```python
from build123d import *

# Parameters (mm, degrees)
SKETCH1_R           = 40
BOSS_EXTRUDE1_DEPTH = 30
FILLET1_R           = 5
SKETCH2_R           = 36
CUT_EXTRUDE1_DEPTH  = 25


with BuildPart() as part:
    # Sketch1 → Boss-Extrude1 (new body)
    with BuildSketch(Plane(origin=(0, 0, 0), x_dir=(1, 0, 0), z_dir=(0, 1, 0))):
        with Locations(Location((0, 0, 0), (0, 0, 270))):
            Circle(SKETCH1_R)
    extrude(amount=BOSS_EXTRUDE1_DEPTH)

    # Fillet1
    fillet1_edges = [part.edges().sort_by_distance(p)[0] for p in [
        (0, 30, -40),
    ]]
    fillet(fillet1_edges, radius=FILLET1_R)

    # Sketch2 → Cut-Extrude1 (cut)
    with BuildSketch(Plane.XZ):
        with Locations(Location((0, 0, 0), (0, 0, 270))):
            Circle(SKETCH2_R)
    extrude(amount=-CUT_EXTRUDE1_DEPTH, mode=Mode.SUBTRACT)


solid = part.part
```
CAD build for the part. Positions are in the model's coordinates, mm. A direction names the side the tool comes from. Round coordinates to 2 decimals unless told otherwise and drop trailing zeros. Order: outer loops, then holes, each group sorted by start corner. A loop starts at its lowest first (then second) coordinate and runs counter-clockwise, first axis right, second up.
Item 1: Saw through at A-A on z = 0. Write the cut outline in (x, y).
Item 2: Pin check, flat tips, straight feed: pin 1 (4 mm diameter, centred on x = -8.5, y = 24.5, fed in from +Z); pin 2 (5 mm diameter, centred on y = 10, z = 3, fed in from +X); pin 3 (1 mm diameter, centred on x = -15, y = 14, fed in from +Z); pin 4 (6 mm diameter, centred on x = 0, y = 25.5, fed in from +Z). Stop position of each tip, or through.
Item 3: Probe line 1 along X through (y, z) = (19.5, 0); line 2 along Y through (x, z) = (7, 15); line 3 along X through (y, z) = (8.25, -12). List the from-to ranges inside material, lowest first.
Item 4: Saw through at B-B on x = 0. Write the cut outline in (y, z), then the cut area to 3 significant figures.
Item 5: Saw through at C-C on y = 11.25. Write the cut outline in (x, z), then the cut area to 3 significant figures.
Item 6: Saw through at D-D on y = 26.75. Write the cut outline in (x, z), then the cut area to 3 significant figures.
Item 7: Mould opens along X. For faces 3 (the face through (0, 30, 0)), 4 (the face through (1, 25, 1)), 5 (the face through (-39.05, 12.32, -8.67)) say: pulls with the +X half, pulls with the -X half, needs draft (parallel to the pull), parting line crosses it, or undercut.
Item 8: Tool access for faces 1 (the face through (15, 0, -33)), 2 (the face through (10.81, 12.32, -34.34)): list every direction of +Z, -Z, +X, -X, +Y, -Y with a clear straight run to the whole face (end or side of a thin tool).
Reported:
1. outline: (-40, 0) - (-36, 0) - (-36, 25) - (36, 25) - (36, 0) - (40, 0) - (40, 25) arc R5 ccw to (35, 30) - (-35, 30) arc R5 ccw to (-40, 25) - close
2. pin 1: stops at z = 39.47
2. pin 2: stops at x = 40
2. pin 3: stops at z = 37.28
2. pin 4: stops at z = 40
3. line 1: x = -40 to -36, 36 to 40
3. line 2: y = 25 to 30
3. line 3: x = -38.16 to -33.94, 33.94 to 38.16
4. outline: (0, -40) - (25, -40) arc R5 ccw to (30, -35) - (30, 35) arc R5 ccw to (25, 40) - (0, 40) - (0, 36) - (25, 36) - (25, -36) - (0, -36) - close
4. area: 589 mm2
5. outline: circle Ø80 at (0, 0); hole circle Ø72 at (0, 0)
5. area: 955 mm2
6. outline: circle Ø79.37 at (0, 0)
6. area: 4,950 mm2
7. face 3: needs draft
7. face 4: undercut
7. face 5: parting line crosses it
8. face 1: +Z, -Z, +X, -X, -Y
8. face 2: -Y
